Autodesk Inventor part; units mm, degrees
ref_plane "YZ Plane" through (0, 0, 0) normal (1, 0, 0) x (0, 1, 0)
ref_plane "XZ Plane" through (0, 0, 0) normal (0, 1, 0) x (-1, 0, 0)
ref_plane "XY Plane" through (0, 0, 0) normal (0, 0, 1) x (1, 0, 0)
sketch "スケッチ1" plane through (0, 0, 0) normal (0, 0, 1) x (1, 0, 0)
  point P0 (0, 0)
sketch "スケッチ2" plane through (0, 0, 0) normal (0, 0, 1) x (1, 0, 0)
  line L0 (100, -52.5) -> (-100, -52.5)
  line L1 (-100, -52.5) -> (-100, 52.5)
  line L2 (-100, 52.5) -> (100, 52.5)
  line L3 (100, 52.5) -> (100, -52.5)
  line L4 (100, -52.5) -> (-100, 52.5) construction
  line L5 (-100, -52.5) -> (100, 52.5) construction
  circle A0 centre (-48, -32) radius 6.05
  circle A1 centre (48, -32) radius 12.55
  circle A2 centre (48, -32) radius 17.5
  circle A3 centre (65.5, -32) radius 2.05
  circle A4 centre (48, -14.5) radius 2.05
  circle A5 centre (30.5, -32) radius 2.05
  circle A6 centre (48, -49.5) radius 2.05
  circle A7 centre (-48, -32) radius 9
  circle A8 centre (-57, -32) radius 1.6
  circle A9 centre (-48, -41) radius 1.6
  circle A10 centre (-39, -32) radius 1.6
  circle A11 centre (-48, -23) radius 1.6
  line L6 (95, 47.5) -> (-95, 47.5)
  line L7 (-95, 47.5) -> (-95, -47.5)
  line L8 (-95, -47.5) -> (95, -47.5)
  line L9 (95, -47.5) -> (95, 47.5)
  line L10 (-95, 47.5) -> (-95, 22.5) construction
  line L11 (-96.6, 47.5) -> (-96.6, 22.5)
  line L12 (-93.4, 22.5) -> (-93.4, 47.5)
  arc A12 (-93.4, 47.5) -> (-96.6, 47.5) centre (-95, 47.5) ccw
  arc A13 (-96.6, 22.5) -> (-93.4, 22.5) centre (-95, 22.5) ccw
  line L13 (-95, 47.5) -> (-70, 47.5) construction
  line L14 (-95, -47.5) -> (-95, -22.5) construction
  line L15 (-93.4, -47.5) -> (-93.4, -22.5)
  line L16 (-96.6, -22.5) -> (-96.6, -47.5)
  arc A14 (-96.6, -47.5) -> (-93.4, -47.5) centre (-95, -47.5) ccw
  arc A15 (-93.4, -22.5) -> (-96.6, -22.5) centre (-95, -22.5) ccw
  line L17 (-95, -47.5) -> (-70, -47.5) construction
  line L18 (95, 47.5) -> (95, 22.5) construction
  line L19 (96.6, 47.5) -> (96.6, 22.5)
  line L20 (93.4, 22.5) -> (93.4, 47.5)
  arc A16 (93.4, 47.5) -> (96.6, 47.5) centre (95, 47.5) ccw
  arc A17 (96.6, 22.5) -> (93.4, 22.5) centre (95, 22.5) ccw
  line L21 (95, 47.5) -> (120, 47.5) construction
  line L22 (95, -47.5) -> (95, -72.5) construction
  line L23 (93.4, -47.5) -> (93.4, -72.5)
  line L24 (96.6, -72.5) -> (96.6, -47.5)
  arc A18 (96.6, -47.5) -> (93.4, -47.5) centre (95, -47.5) ccw
  arc A19 (93.4, -72.5) -> (96.6, -72.5) centre (95, -72.5) ccw
  line L25 (95, -47.5) -> (120, -47.5) construction
  line L26 (-100, -32) -> (100, -32)
  circle A20 centre (0, -32) radius 9
  circle A21 centre (0, -32) radius 39
  line L27 (-85, 52.5) -> (85, 52.5)
  line L28 (85, 52.5) -> (85, 47.5)
  line L29 (85, 47.5) -> (-85, 47.5)
  line L30 (-85, 47.5) -> (-85, 52.5)
  line L31 (-85, 47.5) -> (0, 0)
  line L32 (0, 0) -> (85, 47.5)
  line L33 (-100, 0) -> (100, 0)
  line L34 (100, 0) -> (100, -62.5)
  line L35 (100, -62.5) -> (-100, -62.5)
  line L36 (-100, -62.5) -> (-100, 0)
  arc A22 (100, 52.5) -> (-100, 52.5) centre (0, 0) ccw
  circle A23 centre (0, 58) radius 12
  line L37 (0, 112.9436) -> (0, -32)
  circle A24 centre (0, 58) radius 9
  circle A25 centre (0, 70) radius 1.55
  circle A26 centre (0, 46) radius 1.55
  line L38 (75, -47.5) -> (-75, -47.5)
  line L39 (-75, -47.5) -> (-75, 22.5)
  line L40 (-75, 22.5) -> (75, 22.5)
  line L41 (75, 22.5) -> (75, -47.5)
  line L42 (75, -47.5) -> (-75, 22.5) construction
  line L43 (-75, -47.5) -> (75, 22.5) construction
  circle A27 centre (-75, 22.5) radius 1.6
  circle A28 centre (75, 22.5) radius 1.6
  circle A29 centre (75, -47.5) radius 1.6
  circle A30 centre (-75, -47.5) radius 1.6
  point P0 (-95, 35)
  point P1 (-95, -35)
  point P2 (95, 35)
  point P3 (95, -60)
  point P4 (-39.1422, -33.5937)
  point P5 (-39.1422, -30.4063)
  point P6 (0, 52.5)
  point P7 (85, 52.5)
  point P8 (48.45, -47.5)
  point P9 (47.55, -47.5)
  point P10 (100, -52.5)
  point P11 (0, -12.5)
  dimension "d9" = 35
  dimension "d15" = 18
  dimension "d0" = 200
  dimension "d1" = 105
  dimension "d5" = 12.1
  dimension "d6" = 25.1
  dimension "d10" = 4.1
  dimension "d13" = 360
  dimension "d16" = 3.2
  dimension "d19" = 360
  dimension "d21" = 5
  dimension "d22" = 25
  dimension "d23" = 90
  dimension "d24" = 3.2
  dimension "d25" = 25
  dimension "d26" = 90
  dimension "d27" = 3.2
  dimension "d28" = 25
  dimension "d29" = 90
  dimension "d30" = 3.2
  dimension "d31" = 25
  dimension "d32" = 90
  dimension "d33" = 3.2
  dimension "d36" = 20.5
  dimension "d37" = 18
  dimension "d38" = 78
  dimension "d39" = 48
  dimension "d40" = 48
  dimension "d43" = 170
  dimension "d44" = 85
  dimension "d46" = 62.5
  dimension "d47" = 24
  dimension "d48" = 90
  dimension "d49" = 18
  dimension "d50" = 3.1
  dimension "d51" = 3.1
  dimension "d52" = 150
  dimension "d53" = 70
  dimension "d54" = 3.2
  dimension "d55" = 3.2
  dimension "d56" = 3.2
  dimension "d57" = 3.2
  dimension "d62" = 105.5
extrude "押し出し1" add sketch "スケッチ2" along normal blind 3 contours L0 L24 A18 L9 L26 L3 | L26 L9 L33 L3 | L0 A21 L8 A2 A6 A29 L23 | L33 L9 A17 L19 A16 L6 L28 L2 L3 | L26 L41 L33 L9 | L9 A18 L8 A29 L41 L26 | L0 A21 L8 | L2 A23 A25 L37 A22 | L33 L41 A28 L40 L32 L6 L20 A17 L9 | L41 A29 L8 A2 A3 L26 | L26 A3 A2 A4 A21 L33 L41 | L0 L1 L26 L16 A14 L8 A30 A21 | A21 A2 L8 | L8 A21 A10 L26 A20 A5 A2 | L28 L6 A23 L2 | L37 A25 A23 L2 A22 | L33 A21 L32 L40 A28 L41 | L26 A2 A3 | A3 A2 L26 | L8 A30 L39 L26 A8 A7 A9 A10 A21 | L8 A6 A2 | A2 A21 A1 L26 A3 L8 A6 | A2 A5 L26 A1 A21 | A23 L6 A26 L37 A24 L2 | L2 A24 L37 A25 A23 | L32 L40 L37 A26 A23 L6 | L2 L30 L6 A12 L11 A13 L7 L33 L1 | A16 L6 L9 | L33 L32 A21 | A21 A2 A5 L26 A20 L37 L33 | A3 L26 A1 A21 A2 A4 | A2 L26 A3 | A3 L26 A2 | L1 L33 L7 A15 L16 L26 | A21 L26 A10 | A10 A7 A21 | A6 L8 A2 | A2 A6 | A6 L8 | A5 L26 A2 | A2 L26 A5 | A21 L26 A1 | A1 L26 A21 | A2 A6 L8 | A23 A26 L6 | L32 A21 L37 L40 | L2 A23 L6 L30 | A25 L37 A24 L2 A23 | A21 A1 L26 A5 A2 | L32 L37 A21 | L33 A21 L31 | L37 A20 L26 A10 A21 L33 | L31 A21 L37 | A4 A2 | A2 A4 | A30 L8 L15 L26 L39 | A10 L26 A7 | A7 A9 A8 L26 A0 A10 | L26 A21 A10 | L26 A10 A7 | A7 A10 A21 | L26 A5 A2 | A2 A5 L26 | A1 A21 L26 | L26 A21 A1 | L37 A26 L6 A23 L2 A24 | L40 L31 L6 A23 A26 L37 | L37 A21 L31 L40 | L33 L39 L26 L15 A15 L7 | L7 A13 L12 L6 L31 L40 A27 L39 L33 | A21 L33 L39 A27 L40 L31 | A21 A10 A7 A11 A8 L26 L39 L33 | L37 L26 A20 | A20 L26 L37 | A9 A7 | A7 A9 | L26 A0 A8 A7 A11 A10 | L26 A20 | L6 A26 A23 | L26 A7 A8 | A8 A7 L26 | L26 A0 | A0 L26 | A11 A7 | A7 A11 | A8 L26 A7 | A7 L26 A8
fillet "フィレット1" radius 4 2 edges at (100, 52.5, 1.5) (-100, 52.5, 1.5)
equation "\"d25\" = d22"
equation "\"d27\" = d24"
equation "\"d28\" = d22"
equation "\"d30\" = d24"
equation "\"d31\" = d22"
equation "\"d33\" = d24"
equation "\"d40\" = d39"
properties part number "aaa_small_plate_arm"
Check sheet for the modelled part. Datum: model origin and axes. Units: mm. Coordinates: 2 decimals unless noted, no trailing zeros. Order: outer loops, then holes, each group sorted by start corner. A loop starts at its lowest first (then second) coordinate and runs counter-clockwise, first axis right, second up. Notation, with made-up numbers: M 73.25,45.25 L 77.25,45.25 A10 ccw 77.25,61.25 Z; hole C 1.5,-26.5 d1. An arc over 180 degrees is marked long. One line per question, with ' | ' between items. Start each with the question number.
Item 1: Sectioned sample at D-D on x = 70. Record the cut outline in (y, z), and give its area (3 significant figures).
Item 2: Sectioned sample at B-B on z = 0.8. Count the separate pieces of the cut face and the enclosed holes in it, and give its area (3 significant figures).
Item 3: Sectioned sample at A-A on y = 58. Record the cut outline in (x, z), and give its area (3 significant figures).
Item 4: Sectioned sample at C-C on x = 36.5. Record the cut outline in (y, z).
Item 5: Material ranges on line 1 (Y direction, x = 0, z = 0.75); line 2 (X direction, y = 28, z = 2.7); line 3 (X direction, y = -47.5, z = 2.4), recorded low to high.
Item 6: Gauge pin test, flat ends, axial feed: P1, Ø1.9, axis at x = 75, y = 22.5, coming from the -Z side; P2, Ø1, axis at y = 71, z = 0.5, coming from the -X side; P3, Ø1, axis at y = 62.5, z = 2.5, coming from the -X side. Record the tip position at first contact, or that the pin passes through.
Answer below:
1) outline: M -52.5,0 L 88.64,0 L 88.64,3 L -52.5,3 Z | area: 423 mm^2
2) separate pieces: 1 | enclosed holes: 10 | area: 29,100 mm^2
3) outline: M -96.91,0 L -9,0 L -9,3 L -96.91,3 Z; M 9,0 L 96.91,0 L 96.91,3 L 9,3 Z | area: 527 mm^2
4) outline: M -52.5,0 L 106.88,0 L 106.88,3 L -52.5,3 Z
5) line 1: y = -52.5 to 44.45, 47.55 to 49, 67 to 68.45, 71.55 to 112.94 | line 2: x = -100 to -96.6, -93.4 to 93.4, 96.6 to 100 | line 3: x = -100 to -96.6, -93.4 to -76.6, -73.4 to 73.4, 76.6 to 93.4, 96.6 to 100
6) P1: passes through | P2: stops at x = -88.24 | P3: stops at x = -94.4
